Autodesk Inventor part; units mm, degrees
ref_plane "YZ Plane" through (0, 0, 0) normal (1, 0, 0) x (0, 1, 0)
ref_plane "XZ Plane" through (0, 0, 0) normal (0, 1, 0) x (-1, 0, 0)
ref_plane "XY Plane" through (0, 0, 0) normal (0, 0, 1) x (1, 0, 0)
ref_plane "Work Plane1" through (-1.4224, 0, 0) normal (0, 0, 1) x (1, 0, 0)
sketch "Sketch1" plane through (-1.4224, 0, 0) normal (0, 0, 1) x (1, 0, 0)
  circle A0 centre (280.3224, 21.9203) radius 2.3114
  circle A1 centre (273.9724, 28.2703) radius 2.3114
  circle A2 centre (286.6724, 28.2703) radius 2.3114
  circle A3 centre (278.9, -7.4485) radius 2.3114
  circle A4 centre (273.9724, 15.5703) radius 2.3114
  circle A5 centre (286.6724, 15.5703) radius 2.3114
  arc A6 (292.5755, 18.5809) -> (267.804, 19.7807) centre (280.3224, 21.9203) ccw
  arc A7 (272.6408, -8.5183) -> (285.0265, -9.1182) centre (278.9, -7.4485) ccw
  line L0 (285.0265, -9.1182) -> (292.5755, 18.5809)
  line L1 (272.6408, -8.5183) -> (267.804, 19.7807)
  circle A8 centre (280.3224, 21.9203) radius 2.3114
  circle A9 centre (273.9724, 15.5703) radius 2.3114
  circle A10 centre (286.6724, 15.5703) radius 2.3114
  point P0 (1.4224, 0)
  dimension "d0" = 25.4
  dimension "d1" = 12.7
extrude "Extrusion1" add sketch "Sketch1" along normal blind 1.5875 contours A0 | L0 A7 L1 A6
sketch "Sketch2" plane through (-1.4224, 0, 1.5875) normal (0, 0, 1) x (1, 0, 0)
  point P0 (1.4224, 0)
sketch "Sketch3" plane through (-1.4224, 0, 1.5875) normal (0, 0, 1) x (1, 0, 0)
  circle A0 centre (278.9, -7.4485) radius 2.3114
  circle A1 centre (278.9, -7.4485) radius 3.175
  point P0 (1.4224, 0)
  dimension "d4" = 6.35
sketch "Sketch4" plane through (-1.4224, 0, 1.5875) normal (0, 0, 1) x (1, 0, 0)
  point P0 (1.4224, 0)
sketch "Sketch5" plane through (-1.4224, 0, 1.5875) normal (0, 0, 1) x (1, 0, 0)
  circle A0 centre (273.9724, 28.2703) radius 2.3114
  circle A1 centre (273.9724, 28.2703) radius 2.3114
  circle A2 centre (286.6724, 28.2703) radius 2.3114
  circle A3 centre (286.6724, 15.5703) radius 2.3114
  circle A4 centre (273.9724, 15.5703) radius 2.3114
  line L0 (273.9724, 28.2703) -> (286.6724, 15.5703)
  line L1 (286.6724, 15.5703) -> (286.6724, 28.2703)
  line L2 (286.6724, 28.2703) -> (273.9724, 15.5703)
  circle A5 centre (280.3224, 21.9203) radius 2.2479
  point P0 (1.4224, 0)
  dimension "d5" = 4.4958
extrude "Extrusion2" cut sketch "Sketch3" against normal blind 1.5875 contours A0 | A1
extrude "Extrusion3" cut sketch "Sketch5" against normal blind 1.5875 contours A5 L2 L0 | L0 L2 A5 | L2 A5 L0 | L0 A5 L2
properties part number "raised gear"
Build history of the part. All positions in model axes, mm. Give positions to 0.01 mm unless a question says otherwise; leave off trailing zeros. Loops run counter-clockwise (first coordinate to the right, second up) from the corner with the lowest first, then second, coordinate; pieces in that order, holes last. Notation, with made-up numbers: (37, -6) -> (79, -6) arc R17 ccw to (79, 18) -> close; hole circle Ø8 at (-21, 70). An arc over 180 degrees is marked (long way). Answer in a Markdown table with one row per item.
Item 1: Flat gauge pins, fed straight in: P1, Ø6, axis at x = 269, y = 29, coming from the -Z side; P2, Ø4, axis at x = 272.55, y = 15.57, coming from the +Z side. Where does each tip first touch, or does it go through?
Findings below:
| item | result |
|---|---|
| P1 | stops at z = 0 |
| P2 | passes through |
Item 2: Slice it at B-B on z = 1.05. Give the number of separate pieces and of enclosed holes in the cut face, plus the area to 3 significant figures.
Findings below:
| item | result |
|---|---|
| separate pieces | 1 |
| enclosed holes | 6 |
| area | 775 mm² |
Item 3: Slice it at A-A on x = 272.55. Write the cut outline in (y, z), plus the area to 3 significant figures.
Findings below:
| item | result |
|---|---|
| outline | (-11.45, 0) -> (13.26, 0) -> (13.26, 1.59) -> (-11.45, 1.59) -> close; (17.88, 0) -> (25.96, 0) -> (25.96, 1.59) -> (17.88, 1.59) -> close; (30.58, 0) -> (32.92, 0) -> (32.92, 1.59) -> (30.58, 1.59) -> close |
| area | 55.8 mm² |
Item 4: Slice it at D-D on x = 275.5. Write the cut outline in (y, z), plus the area to 3 significant figures.
Findings below:
| item | result |
|---|---|
| outline | (-13.48, 0) -> (-9.93, 0) -> (-9.93, 1.59) -> (-13.48, 1.59) -> close; (-4.96, 0) -> (34.16, 0) -> (34.16, 1.59) -> (-4.96, 1.59) -> close |
| area | 67.7 mm² |
Item 5: Mould opens along X. For faces 1 (the cylindrical face through (286.32, 30.32, 0.78)), 2 (the flat face through (287.326, 4.537, 0.783)), 3 (the cylindrical face through (277.291, -13.796, 0.783)) say: pulls with the +X half, pulls with the -X half, needs draft (parallel to the pull), parting line crosses it, or undercut.
Findings below:
| item | result |
|---|---|
| face 1 | undercut |
| face 2 | pulls with the +X half |
| face 3 | parting line crosses it |
Item 6: Slice it at C-C on y = 17. Write the cut outline in (x, z).
Findings below:
| item | result |
|---|---|
| outline | (266.86, 0) -> (270.73, 0) -> (270.73, 1.59) -> (266.86, 1.59) -> close; (274.37, 0) -> (283.43, 0) -> (283.43, 1.59) -> (274.37, 1.59) -> close; (287.07, 0) -> (290.72, 0) -> (290.72, 1.59) -> (287.07, 1.59) -> close |
Item 7: Probe line 1 along X through (y, z) = (30, 1.4); line 2 along Y through (x, z) = (274.25, 0.5); line 3 along Y through (x, z) = (278.9, 0.85). List the from-to ranges inside material, lowest first. Write a range as [from, to].
Findings below:
| item | result |
|---|---|
| line 1 | x = [269.1, 271.02], [274.08, 283.72], [286.78, 288.7] |
| line 2 | y = [-12.92, 14], [17.14, 26.7], [29.84, 33.74] |
| line 3 | y = [-13.64, -10.29], [-4.61, 19.67], [24.17, 34.62] |
